Read the model definition and answer for the solid it produces. Units are mm, in the model's axes. A direction names the side the tool comes from. Round coordinates to 2 decimals unless told otherwise and drop trailing zeros. Loops run counter-clockwise (first coordinate to the right, second up) from the corner with the lowest first, then second, coordinate; pieces in that order, holes last. Notation, with made-up numbers: M 0.5,13.5 L 5.5,13.5 A11 cw 5.5,27.5 Z; hole C 60,31 d3. An arc over 180 degrees is marked long. Write each question's results on one line, items separated by ' | '.
```python
from build123d import *

# Parameters (mm, degrees)
F0_W     = 50
F0_H     = 50
F0_R     = 1.5
F1_DEPTH = 2
F3_DEPTH = 25
F4_R     = 2.5
F4_R_2   = 1.5
F5_DEPTH = 2.1


with BuildPart() as f1:
    # F0 (on Top) → F1 (new body)
    with BuildSketch(Plane.XY):
        Rectangle(F0_W, F0_H)
        with Locations((-20.885, -20.885)):
            Circle(F0_R, mode=Mode.SUBTRACT)
        with Locations((0, -21.913239149)):
            Circle(F0_R, mode=Mode.SUBTRACT)
        with Locations((20.885, -20.885)):
            Circle(F0_R, mode=Mode.SUBTRACT)
        with Locations((-21.913239149, 0)):
            Circle(F0_R, mode=Mode.SUBTRACT)
        with Locations((-20.885, 20.885)):
            Circle(F0_R, mode=Mode.SUBTRACT)
        with Locations((21.913239149, 0)):
            Circle(F0_R, mode=Mode.SUBTRACT)
        with Locations((0, 21.913239149)):
            Circle(F0_R, mode=Mode.SUBTRACT)
        with Locations((20.885, 20.885)):
            Circle(F0_R, mode=Mode.SUBTRACT)
    extrude(amount=F1_DEPTH)

    # F2 (on face) → F3 (cut)
    with BuildSketch(Plane.XY.offset(2)):
        with BuildLine():
            ThreePointArc((0, 17.7539922297), (-8.8769961149, 21.470552283), (-17.7539922297, 17.7539922297))
            ThreePointArc((-17.7539922297, 17.7539922297), (-22.8434548265, 8.8769961149), (-17.7539922297, 0))
            ThreePointArc((-17.7539922297, 0), (-22.8434548265, -8.8769961149), (-17.7539922297, -17.7539922297))
            ThreePointArc((-17.7539922297, -17.7539922297), (-8.8769961149, -21.470552283), (0, -17.7539922297))
            ThreePointArc((0, -17.7539922297), (8.8769961149, -21.470552283), (17.7539922297, -17.7539922297))
            ThreePointArc((17.7539922297, -17.7539922297), (22.8434548265, -8.8769961149), (17.7539922297, 0))
            ThreePointArc((17.7539922297, 0), (22.8434548265, 8.8769961149), (17.7539922297, 17.7539922297))
            ThreePointArc((17.7539922297, 17.7539922297), (8.8769961149, 21.470552283), (0, 17.7539922297))
        make_face()
    extrude(amount=-F3_DEPTH, mode=Mode.SUBTRACT)

    # F4 (on face) → F5 (join)
    with BuildSketch(Plane(origin=(0, 0, 0), x_dir=(1, 0, 0), z_dir=(0, 0, -1))):
        with Locations((-20.885, 20.885)):
            Circle(F4_R)
        with Locations((-20.885, 20.885)):
            Circle(F4_R_2, mode=Mode.SUBTRACT)
        with Locations((20.885, 20.885)):
            Circle(F4_R)
        with Locations((20.885, 20.885)):
            Circle(F4_R_2, mode=Mode.SUBTRACT)
        with Locations((20.885, -20.885)):
            Circle(F4_R)
        with Locations((20.885, -20.885)):
            Circle(F4_R_2, mode=Mode.SUBTRACT)
        with Locations((-20.885, -20.885)):
            Circle(F4_R)
        with Locations((-20.885, -20.885)):
            Circle(F4_R_2, mode=Mode.SUBTRACT)
    extrude(amount=F5_DEPTH)


solid = f1.part
```
1. Find section C-C, the plane y = -15.5. Give the vertices of the cut face in (x, z).
Completed:
outline: M -25,0 L -20.43,0 L -20.43,2 L -25,2 Z; M 20.43,0 L 25,0 L 25,2 L 20.43,2 Z
2. Which of the six approach directions +Z, -Z, +X, -X, +Y, -Y give full straight-line access (tool end or side, diameter ignored) to faces 4 (the face through (22.842, 8.727, 1.014)), 5 (the face through (21, -19, -2.1)), 6 (the face through (-22.73, -22.57, -1.04))?
Completed:
face 4: +Z, -Z | face 5: -Z, +X, -X, +Y, -Y | face 6: -Z
3. Find section B-B, the plane x = 8.5. Give the vertices of the cut face in (y, z).
Completed:
outline: M -25,0 L -21.46,0 L -21.46,2 L -25,2 Z; M 21.46,0 L 25,0 L 25,2 L 21.46,2 Z
4. Find section A-A, the plane z = -0.6. Give the vertices of the cut face in (x, y) (3 decimals).
Completed:
outline: C -20.885,-20.885 d5; C -20.885,20.885 d5; C 20.885,-20.885 d5; C 20.885,20.885 d5; hole C -20.885,-20.885 d3; hole C -20.885,20.885 d3; hole C 20.885,-20.885 d3; hole C 20.885,20.885 d3
5. Determine the mould class of faces 1 (the face through (-0.2, 23.4, 1)), 2 (the face through (-19, 21, -2.1)), 3 (the face through (0, -25, 1)) for opening direction Y: released by +Y, released by -Y, zero draft, split by the parting line, or undercut.
Completed:
face 1: undercut | face 2: zero draft | face 3: released by -Y
6. Find the intervals of material crossed by L1, parallel to Y at x = 19, z = 1.65; L2, parallel to X at y = 20, z = -1.9; L3, parallel to X at y = 21.5, z = 1.1, in increasing order.
Completed:
L1: y = -25 to -16.9, -0.86 to 0.86, 16.9 to 25 | L2: x = -23.22 to -22.1, -19.67 to -18.55, 18.55 to 19.67, 22.1 to 23.22 | L3: x = -25 to -22.25, -19.52 to -1.44, 1.44 to 19.52, 22.25 to 25
